The listing builds one solid part. Answer for the finished solid, in the listing's coordinates (mm). Face numbers are marked on the shaded views. A direction names the side the tool comes from. Round coordinates to 2 decimals unless told otherwise and drop trailing zeros. Loops run counter-clockwise (first coordinate to the right, second up) from the corner with the lowest first, then second, coordinate; pieces in that order, holes last. Notation, with made-up numbers: (13, 8) -> (67, 8) arc R10 cw to (67, 23) -> close; hole circle Ø10 at (-26, 68). An arc over 180 degrees is marked (long way). Write each question's results on one line, items separated by ' | '. Start each with the question number.
(1) Flat-ended cylindrical pins translate along their axes: pin 1 (3 mm diameter, centred on y = 28, z = 3, fed in from -X); pin 2 (3 mm diameter, centred on y = 22.5, z = 4, fed in from +X). Find the tip coordinate at first contact, or state that the pin passes through.
(2) The part is cut by section B-B (y = 26.5). Determine the outline of the cut face in (x, z).
(3) The part is cut by section C-C (z = 3.3). Determine the outline of the cut face in (x, y).
(4) For the marked faces 1, 2 and 3, determine the directions among +Z, -Z, +X, -X, +Y, -Y from which every point of the face is accessible in a straight line to the end or side of a thin tool.
(5) Determine the mould class of the marked faces 4, 5, 6 and 7 for opening direction Y: released by +Y, released by -Y, zero draft, split by the parting line, or undercut.
(6) Straight lines are drawn through the part: probe 1 along Y at (x, z) = (4, 3.85); probe 2 along X at (y, z) = (42.5, 3.5); probe 3 along Y at (x, z) = (8.75, 1.8). For each, find the intervals that lie inside material, in ascending order.
(7) The part is cut by section A-A (x = 14.75). Determine the outline of the cut face in (y, z), plus the area to 3 significant figures.
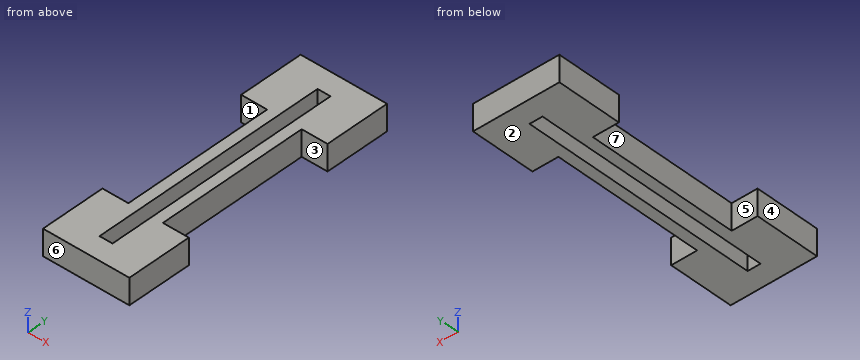
```python
from build123d import *

# Parameters (mm, degrees)
SKETCH1_W           = 3
SKETCH1_H           = 55
BOSS_EXTRUDE1_DEPTH = 6


with BuildPart() as part:
    # Sketch1 → Boss-Extrude1 (new body)
    with BuildSketch(Plane.XY):
        Polygon((0, 0), (20, 0), (20, 15), (14, 15), (14, 50), (20, 50), (20, 65), (0, 65), (0, 50), (6, 50), (6, 15), (0, 15), align=None)
        with Locations((10, 32.5)):
            Rectangle(SKETCH1_W, SKETCH1_H, mode=Mode.SUBTRACT)
    extrude(amount=BOSS_EXTRUDE1_DEPTH)


solid = part.part
```
Checked values:
1) pin 1: stops at x = 6 | pin 2: stops at x = 14
2) outline: (6, 0) -> (8.5, 0) -> (8.5, 6) -> (6, 6) -> close; (11.5, 0) -> (14, 0) -> (14, 6) -> (11.5, 6) -> close
3) outline: (0, 0) -> (20, 0) -> (20, 15) -> (14, 15) -> (14, 50) -> (20, 50) -> (20, 65) -> (0, 65) -> (0, 50) -> (6, 50) -> (6, 15) -> (0, 15) -> close; hole (8.5, 5) -> (11.5, 5) -> (11.5, 60) -> (8.5, 60) -> close
4) face 1: +Z, -Z, -X | face 2: -Z, +X, -X, +Y, -Y | face 3: +Z, -Z, +X
5) face 4: zero draft | face 5: undercut | face 6: released by -Y | face 7: undercut
6) probe 1: y = 0 to 15, 50 to 65 | probe 2: x = 6 to 8.5, 11.5 to 14 | probe 3: y = 0 to 5, 60 to 65
7) outline: (0, 0) -> (15, 0) -> (15, 6) -> (0, 6) -> close; (50, 0) -> (65, 0) -> (65, 6) -> (50, 6) -> close | area: 180 mm2
